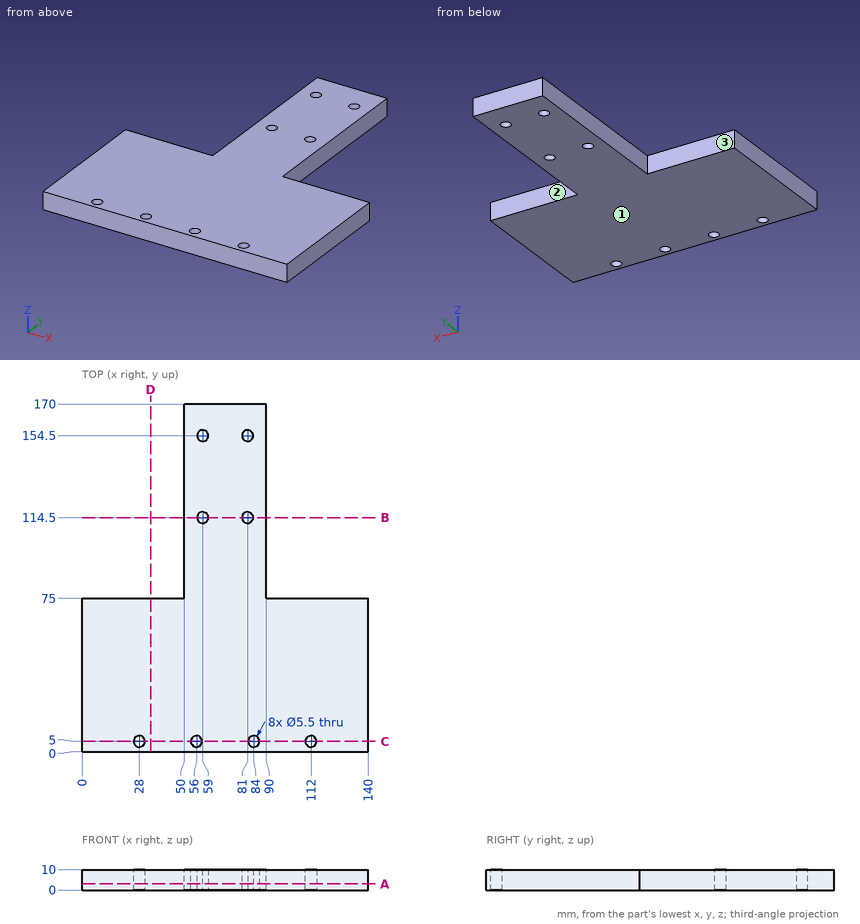
For this review, use the dimensioned drawing (mm, ordinates from the lowest corner) and the shaded views. A direction names the side the tool comes from. Give positions to 0.01 mm unless a question says otherwise; leave off trailing zeros. Order: outer loops, then holes, each group sorted by start corner. A loop starts at its lowest first (then second) coordinate and runs counter-clockwise, first axis right, second up. Notation, with made-up numbers: M 42.25,54 L 65.25,54 A13 ccw 65.25,74 Z; hole C -33.5,12 d7. An arc over 180 degrees is marked long. Use one line per item in the form item = value. Start each with the question number.
Item 1: We need section C-C on y = 5. Give the boundary of the cut face in (x, z).
Item 2: We need section B-B on y = 114.5. Give the boundary of the cut face in (x, z).
Item 3: We need section A-A on z = 3. Give the number of separate pieces and of enclosed holes in the cut face, plus the area to 3 significant figures.
Item 4: We need section D-D on x = 33.5. Give the boundary of the cut face in (y, z), plus the area to 3 significant figures.
Item 5: Insertion check: pin 1 Ø3.5 at (x, y) = (59, 154.5) entering from -Z; pin 2 Ø3 at (y, z) = (102.5, 4.5) entering from -X; pin 3 Ø5 at (y, z) = (145, 6) entering from +X; pin 4 Ø3 at (x, z) = (32, 3) entering from +Y. Each pin has a flat end and moves straight along its axis. Give the tip position at first contact, or say it passes through.
Item 6: For the marked faces 1, 2 and 3, list the 3-axis set-ups (+Z, -Z, +X, -X, +Y, -Y) from which the entire face can be reached by the end or side of a thin tool; tool diameter is ignored.
Item 7: To check wall thickness, follow line 1 along Y through (x, z) = (59, 2.5); line 2 along Y through (x, z) = (56, 3); line 3 along X through (y, z) = (154.5, 7.25). State the ranges of each line that lie inside material, in increasing order. Write a range as from..to.
Completed:
q1.outline = M 0,0 L 25.25,0 L 25.25,10 L 0,10 Z; M 30.75,0 L 53.25,0 L 53.25,10 L 30.75,10 Z; M 58.75,0 L 81.25,0 L 81.25,10 L 58.75,10 Z; M 86.75,0 L 109.25,0 L 109.25,10 L 86.75,10 Z; M 114.75,0 L 140,0 L 140,10 L 114.75,10 Z
q2.outline = M 50,0 L 56.25,0 L 56.25,10 L 50,10 Z; M 61.75,0 L 78.25,0 L 78.25,10 L 61.75,10 Z; M 83.75,0 L 90,0 L 90,10 L 83.75,10 Z
q3.separate_pieces = 1
q3.enclosed_holes = 8
q3.area = 14,100 mm²
q4.outline = M 0,0 L 75,0 L 75,10 L 0,10 Z
q4.area = 750 mm²
q5.pin_1 = through
q5.pin_2 = 50
q5.pin_3 = 90
q5.pin_4 = 75
q6.face_1 = -Z, +X, -X, +Y, -Y
q6.face_2 = +Z, -Z, +X, +Y
q6.face_3 = +Z, -Z, -X, +Y
q7.line_1 = 0..111.75, 117.25..151.75, 157.25..170
q7.line_2 = 0..2.25, 7.75..170
q7.line_3 = 50..56.25, 61.75..78.25, 83.75..90
